Input: part model. Units: mm. Frame: model coordinates. A direction names the side the tool comes from. Round coordinates to 2 decimals unless told otherwise and drop trailing zeros. Write each loop counter-clockwise with the first axis right and the second up, starting at its lowest first coordinate (ties: lowest second). Pieces come first, ordered by that corner, then holes. Notation, with made-up numbers: M 9,15.25 L 33,15.25 A18 cw 33,46.25 Z; hole C 18,-28 d4. An arc over 180 degrees is marked long. Write each question's results on one line, items separated by ' | '. Start each with the question number.
```python
from build123d import *

# Parameters (mm, degrees)
SKETCH1_W           = 37.589281877
SKETCH1_H           = 10
BOSS_EXTRUDE1_DEPTH = 33.4
SKETCH2_R           = 6.5
CUT_EXTRUDE1_DEPTH  = 10
SKETCH3_R           = 1.6
CUT_EXTRUDE2_DEPTH  = 50
SKETCH4_R           = 6.6
SKETCH4_R_2         = 2.75
BOSS_EXTRUDE2_DEPTH = 2


with BuildPart() as part:
    # Sketch1 → Boss-Extrude1 (new body)
    with BuildSketch(Plane.XY):
        with Locations((10.006008035, 10.584218221)):
            Rectangle(SKETCH1_W, SKETCH1_H)
    extrude(amount=BOSS_EXTRUDE1_DEPTH)

    # Sketch2 → Cut-Extrude1 (cut)
    with BuildSketch(Plane(origin=(0, 15.584218221, 0), x_dir=(1, 0, 0), z_dir=(0, 1, 0))):
        with Locations(Location((6.211367096, -24.9, 0), (0, 0, 270))):
            Circle(SKETCH2_R)
    extrude(amount=-CUT_EXTRUDE1_DEPTH, mode=Mode.SUBTRACT)

    # Sketch3 → Cut-Extrude2 (cut)
    with BuildSketch(Plane.XY.offset(33.4)):
        with Locations((-3.288632904, 10.584218221)):
            Circle(SKETCH3_R)
        with Locations((22.800648973, 10.584218221)):
            Circle(SKETCH3_R)
    extrude(amount=-CUT_EXTRUDE2_DEPTH, mode=Mode.SUBTRACT)

    # Sketch4 → Boss-Extrude2 (add)
    with BuildSketch(Plane.XZ.offset(-5.584218221)):
        with Locations((6.211367096, 24.9)):
            Circle(SKETCH4_R)
        with Locations(Location((6.211367096, 24.9, 0), (0, 0, 270))):
            Circle(SKETCH4_R_2, mode=Mode.SUBTRACT)
    extrude(amount=-BOSS_EXTRUDE2_DEPTH)


with BuildPart() as body_2:
    # Mirror1: mirrored copy
    add(part.part.mirror(Plane(origin=(-8.788632904, 15.584218221, 33.4), x_dir=(0, 0, 1), z_dir=(0, 1, 0))))


solid = body_2.part
```
1. Access query for faces 5 (the face through (24.327, 20.104, 16.934)), 6 (the face through (3.722, 19.528, 30.904)). Directions: +Z, -Z, +X, -X, +Y, -Y. A direction counts if a zero-diameter tool reaches every point of the face in a straight line with its end or side. Return the directions, or none.
2. Contact query for flat-ended pins moving along their axis: P1, Ø3.5, axis at x = -3.29, y = 20.58, coming from the -Z side; P2, Ø4, axis at x = 8.5, z = 22.5, coming from the -Y side. Output: stop coordinate, or through.
3. Line query: L1, parallel to X at y = 20, z = 27; L2, parallel to X at y = 20, z = 5.5; L3, parallel to Z at x = 6, y = 18.75. Output: solid intervals per line, ascending. Write a range as from..to.
4. Draft query along Z for faces 1 (the face through (6, 23.584, 22)), 2 (the face through (28.801, 21, 16)), 3 (the face through (10, 21, 0)), 4 (the face through (10, 21, 33.4)). Return one class per face: +Z half, -Z half, draft (parallel to the pull), parting line (faces both ways), or undercut.
5. Cut plane B-B on y = 21.75. Output: boundary loops of the cut face in (x, z), and give its area (3 significant figures).
6. Cut plane A-A on z = 24.9. Output: boundary loops of the cut face in (x, y), and give its area (3 significant figures).
7. Cut plane D-D on y = 17.5. Output: boundary loops of the cut face in (x, z), and give its area (3 significant figures).
8. Cut plane C-C on z = 30. Output: boundary loops of the cut face in (x, y), and give its area (3 significant figures).
Answers follow:
1) face 5: +Z, -Z | face 6: -Y
2) P1: stops at z = 0 | P2: stops at y = 23.58
3) L1: x = -8.79..-4.78, -1.8..0.06, 12.36..21.31, 24.29..28.8 | L2: x = -8.79..-4.78, -1.8..21.31, 24.29..28.8 | L3: z = 0..18.4, 31.4..33.4
4) face 1: undercut | face 2: draft | face 3: -Z half | face 4: +Z half
5) outline: M -8.79,0 L -4.38,0 L -4.38,33.4 L -8.79,33.4 Z; M -2.19,0 L 21.7,0 L 21.7,33.4 L -2.19,33.4 Z; M 23.9,0 L 28.8,0 L 28.8,33.4 L 23.9,33.4 Z; hole C 6.21,24.9 d13 | area: 976 mm2
6) outline: M -8.79,15.58 L -0.29,15.58 L -0.29,23.58 L 3.46,23.58 L 3.46,25.58 L -8.79,25.58 Z; M 8.96,23.58 L 12.71,23.58 L 12.71,15.58 L 28.8,15.58 L 28.8,25.58 L 8.96,25.58 Z; hole C -3.29,20.58 d3.2; hole C 22.8,20.58 d3.2 | area: 245 mm2
7) outline: M -8.79,0 L 28.8,0 L 28.8,33.4 L -8.79,33.4 Z; hole C 6.21,24.9 d13 | area: 1,120 mm2
8) outline: M -8.79,15.58 L 2.18,15.58 L 2.18,23.58 L 10.24,23.58 L 10.24,15.58 L 28.8,15.58 L 28.8,25.58 L -8.79,25.58 Z; hole C -3.29,20.58 d3.2; hole C 22.8,20.58 d3.2 | area: 295 mm2
